Source: CAD feature listing. Evaluate the final solid. Frame: model axes, mm. Face numbers are marked on the shaded views. A direction names the side the tool comes from. Give positions to 0.01 mm unless a question says otherwise; leave off trailing zeros. Order: outer loops, then holes, each group sorted by start corner. A loop starts at its lowest first (then second) coordinate and runs counter-clockwise, first axis right, second up.
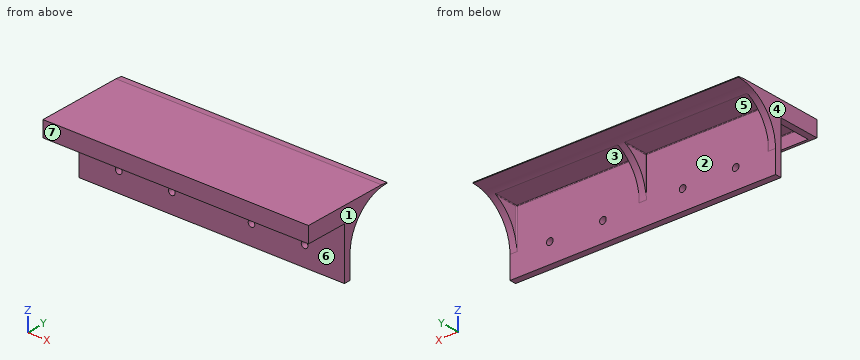
from build123d import *

# Parameters (mm, degrees)
F0_W      = 200
F0_H      = 50
F0_H_2    = 1
F1_DEPTH  = 70
F2_W      = 32
F2_H      = 39
F3_DEPTH  = 200
F5_DEPTH  = 200
F6_W      = 30
F6_H      = 9
F7_DEPTH  = 195
F8_DEPTH  = 5
F9_START  = -97.5
F9_DEPTH  = 5
F11_START = -5
F10_W     = 28.059584938
F10_H     = 30
F11_DEPTH = 92.5
F12_START = -102.5
F12_DEPTH = 92.5
F13_R     = 2.5
F14_DEPTH = 60
F15_R     = 0.5
F16_SIZE2 = 0.5
F16_SIZE  = 5


with BuildPart() as f1:
    # F0 (on Front) → F1 (new body)
    with BuildSketch(Plane.XZ):
        with Locations((-100, -25)):
            Rectangle(F0_W, F0_H)
        with Locations((-100, 0.5)):
            Rectangle(F0_W, F0_H_2)
    extrude(amount=F1_DEPTH)

    # F2 (on Right) → F3 (cut)
    with BuildSketch(Plane.YZ):
        with Locations((-54, -30.5)):
            Rectangle(F2_W, F2_H)
    extrude(amount=-F3_DEPTH, mode=Mode.SUBTRACT)

    # F4 (on Right) → F5 (cut)
    with BuildSketch(Plane.YZ):
        with BuildLine():
            Line((0, -50), (0, 0))
            ThreePointArc((0, 0), (-23.3345237792, -9.6654762208), (-33, -33))
            Line((-33, -33), (-33, -50))
            Line((-33, -50), (0, -50))
        make_face()
    extrude(amount=-F5_DEPTH, mode=Mode.SUBTRACT)

    # F6 (on Right) → F7 (cut)
    with BuildSketch(Plane.YZ):
        with Locations((-53, -6.5)):
            Rectangle(F6_W, F6_H)
    extrude(amount=-F7_DEPTH, mode=Mode.SUBTRACT)

    # F6 (on Right) → F8 (join)
    with BuildSketch(Plane.YZ):
        with Locations((-53, -6.5)):
            Rectangle(F6_W, F6_H)
    extrude(amount=-F8_DEPTH)

    # F6 (on Right) → F9 (join)
    with BuildSketch(Plane.YZ.offset(F9_START)):
        with Locations((-53, -6.5)):
            Rectangle(F6_W, F6_H)
    extrude(amount=-F9_DEPTH)

    # F10 (on Right) → F11 (cut)
    with BuildSketch(Plane.YZ.offset(F11_START)):
        with Locations((-18.970207531, -18)):
            Rectangle(F10_W, F10_H)
    extrude(amount=-F11_DEPTH, mode=Mode.SUBTRACT)

    # F10 (on Right) → F12 (cut)
    with BuildSketch(Plane.YZ.offset(F12_START)):
        with Locations((-18.970207531, -18)):
            Rectangle(F10_W, F10_H)
    extrude(amount=-F12_DEPTH, mode=Mode.SUBTRACT)

    # F13 (on Front) → F14 (cut)
    with BuildSketch(Plane.XZ):
        with Locations((-30, -35)):
            Circle(F13_R)
        with Locations((-70, -35)):
            Circle(F13_R)
        with Locations((-130, -35)):
            Circle(F13_R)
        with Locations((-170, -35)):
            Circle(F13_R)
    extrude(amount=F14_DEPTH, mode=Mode.SUBTRACT)

    # F15
    f15_edges = [f1.edges().sort_by_distance(p)[0] for p in [
        (-195, -23.373864, -3),
        (-148.75, -33, -3),
        (-195, -33, -18),
        (-97.5, -23.373864, -3),
        (-97.5, -33, -18),
        (-51.25, -33, -3),
        (-102.5, -33, -18),
        (-102.5, -23.373864, -3),
        (-5, -23.373864, -3),
        (-5, -33, -18),
        (-97.5, -53, -2),
        (-51.25, -38, -2),
        (-195, -53, -2),
        (-148.75, -38, -2),
        (-148.75, -68, -2),
        (-102.5, -53, -2),
        (-102.5, -68, -6.5),
        (-195, -68, -6.5),
        (-97.5, -68, -6.5),
        (-5, -68, -6.5),
        (-5, -53, -2),
        (-51.25, -68, -2),
        (-5, -38, -6.5),
        (-2.5, -38, -11),
        (-102.5, -38, -6.5),
        (-100, -38, -11),
        (-197.5, -38, -11),
        (-195, -38, -6.5),
        (-97.5, -38, -6.5),
    ]]
    fillet(f15_edges, radius=F15_R)

    # F16
    f16_edges = [f1.edges().sort_by_distance(p)[0] for p in [
        (-100, 0, 1),
    ]]
    f16_side = f1.faces().sort_by_distance((-100, -35, 1))[0]
    chamfer(f16_edges, length=F16_SIZE, length2=F16_SIZE2, reference=f16_side)


solid = f1.part
1) Section query A-A on x = -70. Output: boundary loops of the cut face in (y, z), and give its area (3 significant figures).
Checks:
outline: (-70, -11) - (-68, -11) - (-68, -2.5) arc R0.5 cw to (-67.5, -2) - (-38.5, -2) arc R0.5 cw to (-38, -2.5) - (-38, -32.5) - (-33, -32.5) - (-33, -3.5) arc R0.5 cw to (-32.5, -3) - (-13.75, -3) arc R33 cw to (0, 0) - (0, 0.5) - (-5, 1) - (-70, 1) - close; (-38, -50) - (-33, -50) - (-33, -37.5) - (-38, -37.5) - close
area: 447 mm2
2) Pull-direction query (X, two-part tool) for the marked faces 1, 2, 3 and 4; classes: +X half, -X half, draft (parallel to the pull), parting line (faces both ways), or undercut.
Checks:
face 1: +X half
face 2: undercut
face 3: undercut
face 4: -X half
3) Section query D-D on x = -105.5. Output: boundary loops of the cut face in (y, z), and give its area (3 significant figures).
Checks:
outline: (-70, -11) - (-68, -11) - (-68, -2.5) arc R0.5 cw to (-67.5, -2) - (-38.5, -2) arc R0.5 cw to (-38, -2.5) - (-38, -50) - (-33, -50) - (-33, -3.5) arc R0.5 cw to (-32.5, -3) - (-13.75, -3) arc R33 cw to (0, 0) - (0, 0.5) - (-5, 1) - (-70, 1) - close
area: 472 mm2
4) Section query C-C on z = -5.5. State how many separate pieces and enclosed holes the cut face has, and give its area (3 significant figures).
Checks:
separate pieces: 1
enclosed holes: 2
area: 2,070 mm2
5) Reachability of the marked faces 5, 6 and 7 from +Z, -Z, +X, -X, +Y, -Y: full face, straight path, thin tool, end or side. Return the list, or none.
Checks:
face 5: -Z, +Y
face 6: -Z
face 7: +Z, -Z, +X, -X, -Y
6) Ray query, L1, parallel to X at y = -45, z = -2.5; L2, parallel to Z at x = -30, y = -35.75; L3, parallel to X at y = -36.65, z = -35. Return the intervals inside material, ascending.
Checks:
L1: x = -200 to -195, -102.5 to -97.5, -5 to 0
L2: z = -50 to -37.5, -32.5 to 1
L3: x = -200 to -172.5, -167.5 to -132.5, -127.5 to -72.5, -67.5 to -32.5, -27.5 to 0
7) Section query B-B on z = -35. Output: boundary loops of the cut face in (x, y), and give its area (3 significant figures).
Checks:
outline: (-200, -38) - (-172.5, -38) - (-172.5, -33) - (-200, -33) - close; (-167.5, -38) - (-132.5, -38) - (-132.5, -33) - (-167.5, -33) - close; (-127.5, -38) - (-72.5, -38) - (-72.5, -33) - (-127.5, -33) - close; (-67.5, -38) - (-32.5, -38) - (-32.5, -33) - (-67.5, -33) - close; (-27.5, -38) - (0, -38) - (0, -33) - (-27.5, -33) - close
area: 900 mm2
8) First-contact query: pin 1 Ø9.5 at (x, y) = (-155.5, -18.5) entering from -Z; pin 2 Ø6 at (x, z) = (-30, -35) entering from +Y; pin 3 Ø8.5 at (x, y) = (-45, -53.5) entering from -Z; pin 4 Ø14 at (y, z) = (-20.5, -10) entering from +X. Flat tips, straight axial feed; report the tip coordinate or a pass-through.
Checks:
pin 1: stops at z = -3
pin 2: stops at y = -33
pin 3: stops at z = -2
pin 4: stops at x = 0
